Can you work these out from the drawing? Everything is in mm from the part's minimum corner. A direction names the side the tool comes from. Coordinates: 2 decimals unless noted, no trailing zeros. Order: outer loops, then holes, each group sorted by start corner. A loop starts at its lowest first (then second) coordinate and runs counter-clockwise, first axis right, second up. Notation, with made-up numbers: (12, 63) -> (43, 63) arc R14 cw to (43, 87) -> close; hole circle Ø10 at (15, -35). An arc over 180 degrees is marked (long way). Put each result on its own line as item: value. Start each with the question number.
Q1. If we section it at B-B (y = 29): Please give me the cut outline in (x, z), and give its area (3 significant figures).
Q2. We'd pull the mould along X, two halves only. Please class the marked faces 1, 2, 3 and 4: +X half, -X half, draft (parallel to the pull), parting line (faces both ways), or undercut.
Q3. If we section it at A-A (z = 10): Please give me the cut outline in (x, y), and give its area (3 significant figures).
Q4. For the marked faces 5 and 6, which set-ups out of +Z, -Z, +X, -X, +Y, -Y let a thin tool reach every point of the face, with its end or its side?
Q5. If we section it at D-D (y = 8): Please give me the cut outline in (x, z), and give its area (3 significant figures).
Q6. Will these pins go through, and if not, where does the flat tip stop? pin 1 (12 mm diameter, centred on x = 41.5, z = 26.5, fed in from -Y); pin 2 (4 mm diameter, centred on x = 21.5, y = 29, fed in from -Z); pin 3 (6 mm diameter, centred on x = 64.5, z = 22, fed in from +Y).
Q7. If we section it at C-C (x = 144): Please give me the cut outline in (y, z), and give its area (4 significant figures).
Q8. Please list where these lines run through material, in increasing order: line 1 along X through (y, z) = (12.5, 19.5); line 2 along Z through (x, y) = (123.5, 4); line 3 along Y through (x, z) = (107, 14).
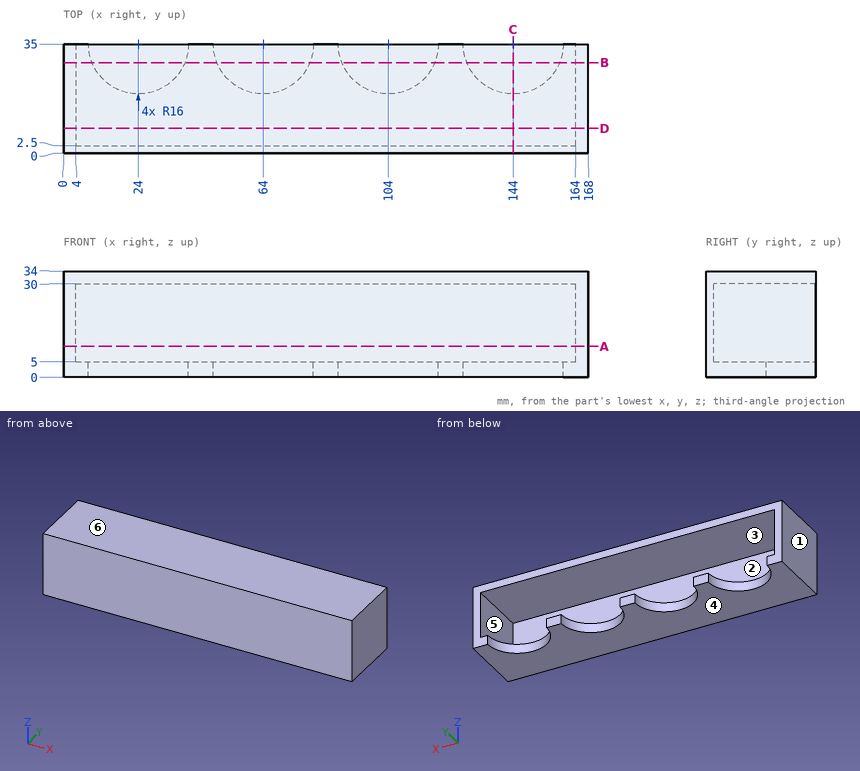
The answers:
1. outline: (0, 0) -> (9.17, 0) -> (9.17, 5) -> (4, 5) -> (4, 30) -> (164, 30) -> (164, 5) -> (158.83, 5) -> (158.83, 0) -> (168, 0) -> (168, 34) -> (0, 34) -> close; (38.83, 0) -> (49.17, 0) -> (49.17, 5) -> (38.83, 5) -> close; (78.83, 0) -> (89.17, 0) -> (89.17, 5) -> (78.83, 5) -> close; (118.83, 0) -> (129.17, 0) -> (129.17, 5) -> (118.83, 5) -> close
1. area: 1,120 mm^2
2. face 1: -X half
2. face 2: undercut
2. face 3: undercut
2. face 4: draft
3. outline: (0, 0) -> (168, 0) -> (168, 35) -> (164, 35) -> (164, 2.5) -> (4, 2.5) -> (4, 35) -> (0, 35) -> close
3. area: 680 mm^2
4. face 5: +Y
4. face 6: +Z, +X, -X, +Y, -Y
5. outline: (0, 0) -> (168, 0) -> (168, 34) -> (0, 34) -> close; hole (4, 5) -> (164, 5) -> (164, 30) -> (4, 30) -> close
5. area: 1,710 mm^2
6. pin 1: y = 0
6. pin 2: z = 30
6. pin 3: y = 2.5
7. outline: (0, 0) -> (19, 0) -> (19, 5) -> (2.5, 5) -> (2.5, 30) -> (35, 30) -> (35, 34) -> (0, 34) -> close
7. area: 297.5 mm^2
8. line 1: 0 to 4, 164 to 168
8. line 2: 0 to 5, 30 to 34
8. line 3: 0 to 2.5
